from build123d import *

# Parameters (mm, degrees)
F0_R     = 8
F0_R_2   = 4
F0_R_3   = 2
F1_DEPTH = 2
F2_DEPTH = 3.7
F3_R     = 1.5


with BuildPart() as f1:
    # F0 (on Top) → F1 (new body)
    with BuildSketch(Plane.XY):
        Circle(F0_R)
        Circle(F0_R_2, mode=Mode.SUBTRACT)
        Circle(F0_R_2)
        Circle(F0_R_3, mode=Mode.SUBTRACT)
        Circle(F0_R_3)
    extrude(amount=F1_DEPTH)

    # F0 (on Top) → F2 (join)
    with BuildSketch(Plane.XY):
        Circle(F0_R_2)
        Circle(F0_R_3, mode=Mode.SUBTRACT)
    extrude(amount=-F2_DEPTH)

    # F3
    f3_edges = [f1.edges().sort_by_distance(p)[0] for p in [
        (-8, 0, 2),
    ]]
    fillet(f3_edges, radius=F3_R)


solid = f1.part
Model file for the job. Use its own axes, mm. Give positions to 0.01 mm unless a question says otherwise; leave off trailing zeros. Write each loop counter-clockwise with the first axis right and the second up, starting at its lowest first coordinate (ties: lowest second). Pieces come first, ordered by that corner, then holes. Notation, with made-up numbers: (67.5, 87.25) -> (112.5, 87.25) arc R11 ccw to (112.5, 96.25) -> close; hole circle Ø4 at (6.25, 16). An arc over 180 degrees is marked (long way). Write item = value, one per line.
(1) Probe line 1 along Y through (x, z) = (0, -2.1); line 2 along Z through (x, y) = (4.5, 2); line 3 along X through (y, z) = (-2, 0.05). List the from-to ranges inside material, lowest first.
Determined:
line_1 = -4 to -2, 2 to 4
line_2 = 0 to 2
line_3 = -7.75 to 7.75
(2) Flat gauge pins, fed straight in: P1, Ø2, axis at x = 3.5, z = -2, coming from the -Y side; P2, Ø3, axis at x = 0, z = -2.5, coming from the +Y side. Where does each tip first touch, or does it go through?
Determined:
P1 = -3.12
P2 = 4
(3) Mould opens along Y. For faces 1 (the face through (-0.867, -3.905, -1.824)), 2 (the face through (0, -2, -2)), 3 (the face through (-4, -2, 0)), 4 (the face through (0, 0, 0)) say: released by +Y, released by -Y, zero draft, split by the parting line, or undercut.
Determined:
face_1 = split by the parting line
face_2 = undercut
face_3 = zero draft
face_4 = undercut
(4) Slice it at A-A, the plane y = 0. Give the cut face in (x, z).
Determined:
outline = (-8, 0) -> (-4, 0) -> (-4, -3.7) -> (-2, -3.7) -> (-2, 0) -> (2, 0) -> (2, -3.7) -> (4, -3.7) -> (4, 0) -> (8, 0) -> (8, 0.5) arc R1.5 ccw to (6.5, 2) -> (-6.5, 2) arc R1.5 ccw to (-8, 0.5) -> close
